from build123d import *

# Parameters (mm, degrees)
SKETCH2_R           = 27.469
BOSS_EXTRUDE1_DEPTH = 4
SKETCH3_R           = 2
CUT_EXTRUDE1_DEPTH  = 5
SKETCH4_R           = 0.5
CUT_EXTRUDE2_DEPTH  = 6


with BuildPart() as part:
    # Sketch2 → Boss-Extrude1 (new body)
    with BuildSketch(Plane(origin=(0, 0, 0), x_dir=(1, 0, 0), z_dir=(0, 1, 0))):
        Circle(SKETCH2_R)
    extrude(amount=BOSS_EXTRUDE1_DEPTH)

    # Sketch3 → Cut-Extrude1 (cut, through all)
    with BuildSketch(Plane(origin=(0, 4, 0), x_dir=(1, 0, 0), z_dir=(0, 1, 0))):
        with Locations((-23.971, 0)):
            Circle(SKETCH3_R)
        with Locations((0, 23.971)):
            Circle(SKETCH3_R)
        with Locations((23.971, 0)):
            Circle(SKETCH3_R)
        with Locations((0, -23.971)):
            Circle(SKETCH3_R)
    extrude(amount=-CUT_EXTRUDE1_DEPTH, mode=Mode.SUBTRACT)

    # Sketch4 → Cut-Extrude2 (cut, through all)
    with BuildSketch(Plane(origin=(0, 5, 0), x_dir=(1, 0, 0), z_dir=(0, 1, 0))):
        Circle(SKETCH4_R)
    extrude(amount=-CUT_EXTRUDE2_DEPTH, mode=Mode.SUBTRACT)


solid = part.part
Source: CAD feature listing. Evaluate the final solid. Frame: model axes, mm. Coordinates: 2 decimals unless noted, no trailing zeros. Loops run counter-clockwise (first coordinate to the right, second up) from the corner with the lowest first, then second, coordinate; pieces in that order, holes last. Notation, with made-up numbers: (-37.75, 14.25) - (-21.75, 14.25) arc R9 cw to (-21.75, 24.25) - close; hole circle Ø9 at (81.5, -31.75). An arc over 180 degrees is marked (long way). One line per question, with ' | ' between items.
1) Section B-B, the plane x = 10. Return loops of the section in (y, z).
Report:
outline: (0, -25.58) - (4, -25.58) - (4, 25.58) - (0, 25.58) - close
2) Line query: line 1 along Z through (x, y) = (0, 2.2); line 2 along Z through (x, y) = (1.5, 2.5). Output: solid intervals per line, ascending.
Report:
line 1: z = -27.47 to -25.97, -21.97 to -0.5, 0.5 to 21.97, 25.97 to 27.47 | line 2: z = -27.43 to -25.29, -22.65 to 22.65, 25.29 to 27.43
3) Section C-C, the plane z = -14.5. Return loops of the section in (x, y).
Report:
outline: (-23.33, 0) - (23.33, 0) - (23.33, 4) - (-23.33, 4) - close
4) Section A-A, the plane y = 2.65. Return loops of the section in (x, z), then the cut area to 3 significant figures.
Report:
outline: circle Ø54.94 at (0, 0); hole circle Ø4 at (-23.97, 0); hole circle Ø4 at (0, -23.97); hole circle Ø4 at (0, 23.97); hole circle Ø1 at (0, 0); hole circle Ø4 at (23.97, 0) | area: 2,320 mm²
5) First-contact query: P1, Ø3.5, axis at x = -23.971, z = 0, coming from the +Y side; P2, Ø6, axis at x = -15.5, z = 5, coming from the -Y side; P3, Ø1, axis at x = -5, y = 3.5, coming from the -Z side; P4, Ø1.5, axis at y = 3, z = -20, coming from the +X side. Flat tips, straight axial feed; report the tip coordinate or a pass-through.
Report:
P1: passes through | P2: stops at y = 0 | P3: stops at z = -27.1 | P4: stops at x = 19.6
6) Pull-direction query (X, two-part tool) for faces 1 (the face through (-0.434, 2.028, -22.019)), 2 (the face through (12.675, 1.972, 24.37)), 3 (the face through (0, 4, 6)), 4 (the face through (22.384, 2.028, 1.217)); classes: released by +X, released by -X, zero draft, split by the parting line, or undercut.
Report:
face 1: undercut | face 2: split by the parting line | face 3: zero draft | face 4: undercut
